Build history of the part. All positions in model axes, mm. Face numbers are marked on the shaded views. A direction names the side the tool comes from. Round coordinates to 2 decimals unless told otherwise and drop trailing zeros. Write each loop counter-clockwise with the first axis right and the second up, starting at its lowest first coordinate (ties: lowest second). Pieces come first, ordered by that corner, then holes. Notation, with made-up numbers: M 89,-38.75 L 147,-38.75 A35 cw 147,-3.75 Z; hole C -36.75,-38.5 d3. An arc over 180 degrees is marked long. Write item = value, one per line.
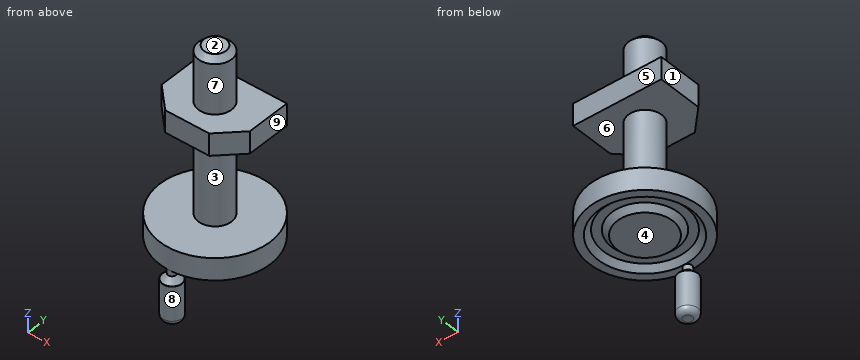
from build123d import *

# Parameters (mm, degrees)
SKETCH_1_R          = 15
EXTRUDE_1_DEPTH     = 150
SKETCH_2_R          = 50
EXTRUDE_2_DEPTH     = 20
SKETCH_3_R          = 42.5
SKETCH_3_R_2        = 25
CUT_EXTRUDE_1_DEPTH = 5
CHAMFER_1_SIZE      = 5
SKETCH_4_R          = 3.75
EXTRUDE_3_DEPTH     = 10
SKETCH_5_R          = 9
EXTRUDE_4_DEPTH     = 36
FILLET_2_R          = 5
CHAMFER_2_SIZE      = 5
CHAMFER_3_SIZE      = 5
SKETCH_6_W          = 80
SKETCH_6_H          = 60
EXTRUDE_5_DEPTH     = 20
CHAMFER_4_SIZE      = 20


with BuildPart() as part:
    # 草图1 → 凸台-拉伸1 (new body)
    with BuildSketch(Plane.XY):
        Circle(SKETCH_1_R)
    extrude(amount=EXTRUDE_1_DEPTH)

    # 草图2 → 凸台-拉伸2 (add)
    with BuildSketch(Plane(origin=(0, 0, 0), x_dir=(-1, 0, 0), z_dir=(0, 0, -1))):
        Circle(SKETCH_2_R)
    extrude(amount=EXTRUDE_2_DEPTH)

    # 草图3 → 切除-拉伸1 (cut)
    with BuildSketch(Plane(origin=(0, 0, -20), x_dir=(-1, 0, 0), z_dir=(0, 0, -1))):
        Circle(SKETCH_3_R)
        Circle(SKETCH_3_R_2, mode=Mode.SUBTRACT)
    extrude(amount=-CUT_EXTRUDE_1_DEPTH, mode=Mode.SUBTRACT)

    # 倒角1
    chamfer_1_edges = [part.edges().sort_by_distance(p)[0] for p in [
        (42.5, 0, -15),
        (25, 0, -15),
    ]]
    chamfer(chamfer_1_edges, length=CHAMFER_1_SIZE - 0.0001)  # a hair under: the kernel refuses the full size

    # 草图4 → 凸台-拉伸3 (add)
    with BuildSketch(Plane(origin=(0, 0, -20), x_dir=(-1, 0, 0), z_dir=(0, 0, -1))):
        with Locations(Location((0, -46.25, 0), (0, 0, 269.999564815))):
            Circle(SKETCH_4_R)
    extrude(amount=EXTRUDE_3_DEPTH)

    # 草图5 → 凸台-拉伸4 (add)
    with BuildSketch(Plane(origin=(0, 0, -30), x_dir=(-1, 0, 0), z_dir=(0, 0, -1))):
        with Locations((0, -46.25)):
            Circle(SKETCH_5_R)
    extrude(amount=EXTRUDE_4_DEPTH)

    # 圆角2
    fillet_2_edges = [part.edges().sort_by_distance(p)[0] for p in [
        (9, -46.25, -66),
    ]]
    fillet(fillet_2_edges, radius=FILLET_2_R)

    # 倒角2
    chamfer_2_edges = [part.edges().sort_by_distance(p)[0] for p in [
        (-2.8483e-05, -42.5, -30),
    ]]
    chamfer(chamfer_2_edges, length=CHAMFER_2_SIZE)

    # 倒角3
    chamfer_3_edges = [part.edges().sort_by_distance(p)[0] for p in [
        (-15, 0, 150),
    ]]
    chamfer(chamfer_3_edges, length=CHAMFER_3_SIZE)

    # 草图6 → 凸台-拉伸5 (add)
    with BuildSketch(Plane.XY.offset(80)):
        Rectangle(SKETCH_6_W, SKETCH_6_H)
    extrude(amount=EXTRUDE_5_DEPTH)

    # 倒角4
    chamfer_4_edges = [part.edges().sort_by_distance(p)[0] for p in [
        (40, -30, 90),
        (-40, -30, 90),
    ]]
    chamfer(chamfer_4_edges, length=CHAMFER_4_SIZE)


solid = part.part
1. Band-saw the part on C-C (z = -7). List the corners of the cut face in (x, y).
Responses:
outline = C 0,0 d100
2. Tool access for the marked faces 5, 6, 7, 8 and 9: list every direction of +Z, -Z, +X, -X, +Y, -Y with a clear straight run to the whole face (end or side of a thin tool).
Responses:
face_5 = +Z, +X, -X, +Y
face_6 = none
face_7 = +Z
face_8 = -Z
face_9 = +Z, +X, +Y, -Y
3. Band-saw the part on B-B (z = 95). List the corners of the cut face in (x, y), plus the area to 3 significant figures.
Responses:
outline = M -40,-10 L -20,-30 L 20,-30 L 40,-10 L 40,30 L -40,30 Z
area = 4,400 mm²
4. Flat gauge pins, fed straight in: pin 1 (5.5 mm diameter, centred on x = -4, y = -42.5, fed in from +Z); pin 2 (5 mm diameter, centred on x = -26, y = 17.5, fed in from +Z); pin 3 (1.5 mm diameter, centred on x = -5, y = 5.5, fed in from -Z); pin 4 (10 mm diameter, centred on y = -20.5, z = 10, fed in from +X). Where does each tip first touch, or does it go through?
Responses:
pin_1 = 0
pin_2 = 100
pin_3 = -20
pin_4 = through
5. Band-saw the part on D-D (z = 16). List the corners of the cut face in (x, y).
Responses:
outline = C 0,0 d30
6. Probe probe 1 along Z at (x, y) = (-18, -25.5); probe 2 along Z at (x, y) = (-18.5, -14); probe 3 along Y at (x, z) = (0, -19). List the from-to ranges inside material, lowest first.
Responses:
probe_1 = -15 to 0, 80 to 100
probe_2 = -20 to 0, 80 to 100
probe_3 = -50 to -41.5, -26 to 26, 41.5 to 50
7. Mould opens along Z. For the marked faces 1, 2, 3 and 4 say: pulls with the +Z half, pulls with the -Z half, needs draft (parallel to the pull), parting line crosses it, or undercut.
Responses:
face_1 = needs draft
face_2 = pulls with the +Z half
face_3 = undercut
face_4 = pulls with the -Z half
